from build123d import *

# Parameters (mm, degrees)
F1_DEPTH = 16
F2_R     = 1.25
F3_R     = 1.25


with BuildPart() as f1:
    # F0 (on Right) → F1 (new body)
    with BuildSketch(Plane.YZ):
        with BuildLine():
            Line((0, -47), (0, 0))
            Line((0, 0), (-3, 0))
            Line((-3, 0), (-3, -31))
            ThreePointArc((-3, -31), (-7.686292, -42.313708), (-19, -47))
            Line((-19, -47), (-35, -47))
            ThreePointArc((-35, -47), (-36.414214, -46.414214), (-37, -45))
            Line((-37, -45), (-37, -40))
            Line((-37, -40), (-40, -40))
            Line((-40, -40), (-40, -47))
            ThreePointArc((-40, -47), (-39.12132, -49.12132), (-37, -50))
            Line((-37, -50), (-3, -50))
            ThreePointArc((-3, -50), (-0.87868, -49.12132), (0, -47))
        make_face()
    extrude(amount=F1_DEPTH)

    # F2
    f2_edges = [f1.edges().sort_by_distance(p)[0] for p in [
        (8, 0, 0),
        (8, -3, 0),
    ]]
    fillet(f2_edges, radius=F2_R)

    # F3
    f3_edges = [f1.edges().sort_by_distance(p)[0] for p in [
        (8, -37, -40),
        (8, -40, -40),
    ]]
    fillet(f3_edges, radius=F3_R)


solid = f1.part
Input: part model. Units: mm. Frame: model coordinates. A direction names the side the tool comes from. Coordinates: 2 decimals unless noted, no trailing zeros. Loops run counter-clockwise (first coordinate to the right, second up) from the corner with the lowest first, then second, coordinate; pieces in that order, holes last. Notation, with made-up numbers: (14.5, -26.75) - (33.5, -26.75) arc R19 cw to (33.5, 4.25) - close; hole circle Ø10 at (50, 57). An arc over 180 degrees is marked (long way). Answer in a Markdown table with one row per item. Add a question column.
Item 1: Access query for faces 4 (the flat face through (8, -3, -16)), 5 (the cylindrical face through (7.89, -39.14, -49.1)), 6 (the flat face through (8, -27, -47)). Directions: +Z, -Z, +X, -X, +Y, -Y. A direction counts if a zero-diameter tool reaches every point of the face in a straight line with its end or side. Return the directions, or none.
Item 2: Section query C-C on y = -28.5. Return the cut outline in (x, z), then the cut area to 3 significant figures.
Item 3: Mould query, pull axis Y, two halves, no side actions, for faces 1 (the cylindrical face through (8.112, -2.624, -0.356)), 2 (the cylindrical face through (8.112, -0.356, -0.376)), 3 (the cylindrical face through (8.112, -37.376, -40.356)). Classes: released by +Y, released by -Y, zero draft, split by the parting line, or undercut.
Item 4: Contact query for flat-ended pins moving along their axis: P1, Ø3, axis at x = 7.5, y = -8.5, coming from the +Z side; P2, Ø4, axis at x = 8.5, y = -21.5, coming from the +Z side; P3, Ø8, axis at x = 11, z = -18, coming from the -Y side. Output: stop coordinate, or through.
Item 5: Line query: line 1 along Y through (x, z) = (3.5, -10.5); line 2 along Z through (x, y) = (4, -30); line 3 along Z through (x, y) = (12, -14.5). Output: solid intervals per line, ascending. Write a range as [from, to].
Item 6: Section query A-A on x = 9.75. Return the cut outline in (y, z).
Item 7: Section query B-B on z = -11.5. Return the cut outline in (x, y).
Recorded:
| question | item | result |
|---|---|---|
| 1 | face 4 | +Z, +X, -X, -Y |
| 1 | face 5 | -Z, +X, -X, -Y |
| 1 | face 6 | +Z, +X, -X |
| 2 | outline | (0, -50) - (16, -50) - (16, -47) - (0, -47) - close |
| 2 | area | 48.0 mm^2 |
| 3 | face 1 | released by -Y |
| 3 | face 2 | released by +Y |
| 3 | face 3 | undercut |
| 4 | P1 | z = -41.58 |
| 4 | P2 | z = -47 |
| 4 | P3 | y = -3 |
| 5 | line 1 | [-3, 0] |
| 5 | line 2 | [-50, -47] |
| 5 | line 3 | [-50, -46.35] |
| 6 | outline | (-40, -47) arc R3 ccw to (-37, -50) - (-3, -50) arc R3 ccw to (0, -47) - (0, -1.25) arc R1.25 ccw to (-1.25, 0) - (-1.75, 0) arc R1.25 ccw to (-3, -1.25) - (-3, -31) arc R16 cw to (-19, -47) - (-35, -47) arc R2 cw to (-37, -45) - (-37, -41.25) arc R1.25 ccw to (-38.25, -40) - (-38.75, -40) arc R1.25 ccw to (-40, -41.25) - close |
| 7 | outline | (0, -3) - (16, -3) - (16, 0) - (0, 0) - close |
